CAD build for the part. Positions are in the model's coordinates, mm. A direction names the side the tool comes from. Coordinates: 2 decimals unless noted, no trailing zeros. Order: outer loops, then holes, each group sorted by start corner. A loop starts at its lowest first (then second) coordinate and runs counter-clockwise, first axis right, second up. Notation, with made-up numbers: (77.5, 72.25) - (136.5, 72.25) arc R15 cw to (136.5, 97.25) - close; hole circle Ø2 at (-0.75, 12). An arc over 180 degrees is marked (long way). Write each question's results on one line, items separated by ' | '. Start each with the question number.
Q1. Wall check: probe 1 along Y at (x, z) = (0, 57); probe 2 along Z at (x, y) = (-16.5, -14); probe 3 along X at (y, z) = (15.5, 40). Give the ranges that are in metal, low to high.
Q2. Pin check, flat tips, straight feed: P1, Ø10, axis at y = -24, z = 52.5, coming from the +X side; P2, Ø2, axis at y = 29.5, z = 26, coming from the -X side; P3, Ø8, axis at y = 28, z = 12, coming from the +X side. Stop position of each tip, or through.
Q3. Which spindle directions (+Z, -Z, +X, -X, +Y, -Y) get a long thin tool onto all of the face, cutting with end or side? Do faces 4 (the flat face through (-1, 1, 0)), 5 (the cylindrical face through (-5.012, 38.172, 47.109)), 6 (the flat face through (-4.447, -38.864, 46.097)). Say none if no direction does.
Q4. Band-saw the part on B-B, the plane y = 0. Write the cut outline in (x, z), then the cut area to 3 significant figures.
Q5. Band-saw the part on A-A, the plane x = 9.5. Write the cut outline in (y, z), then the cut area to 3 significant figures.
Q6. Pull direction Y, two halves, no side cores. Call faces 1 (the flat face through (7.62, -38.18, 40.33)), 2 (the flat face through (-1, 1, 3)), 3 (the cylindrical face through (-5.21, 39.66, 44.37)): released by +Y, released by -Y, zero draft, split by the parting line, or undercut.
Q7. Band-saw the part on D-D, the plane x = 0. Write the cut outline in (y, z).
Q8. Band-saw the part on C-C, the plane z = 82. Write the cut outline in (x, y), then the cut area to 3 significant figures.
```python
from build123d import *

# Parameters (mm, degrees)
SKETCH_R        = 40
PAD_DEPTH       = 90
SKETCH001_R     = 38.5
POCKET_DEPTH    = 87
POCKET001_DEPTH = 50


with BuildPart() as part:
    # Sketch → Pad (new body)
    with BuildSketch(Plane.XY):
        Circle(SKETCH_R)
    extrude(amount=PAD_DEPTH)

    # Sketch001 (on Face3 of Pad) → Pocket (cut)
    with BuildSketch(Plane.XY.offset(90)):
        Circle(SKETCH001_R)
    extrude(amount=-POCKET_DEPTH, mode=Mode.SUBTRACT)

    # Sketch002 → Pocket001 (cut)
    with BuildSketch(Plane.XZ.offset(45)):
        Polygon((-19.683228, 16.045872), (10.932937, 76.430139), (22.858825, 70.387448), (-7.758954, 10), align=None)
    extrude(amount=-POCKET001_DEPTH, mode=Mode.SUBTRACT)


solid = part.part
```
Results below:
1) probe 1: y = -40 to -38.5, 38.5 to 40 | probe 2: z = 0 to 3 | probe 3: x = -36.87 to -35.24, 35.24 to 36.87
2) P1: stops at x = 35.2 | P2: stops at x = -28.07 | P3: stops at x = 32
3) face 4: -Z, +X, -X, +Y, -Y | face 5: +Z | face 6: -Y
4) outline: (-40, 0) - (40, 0) - (40, 90) - (38.5, 90) - (38.5, 3) - (-38.5, 3) - (-38.5, 90) - (-40, 90) - close | area: 501 mm²
5) outline: (-38.86, 0) - (38.86, 0) - (38.86, 90) - (37.31, 90) - (37.31, 3) - (-37.31, 3) - (-37.31, 44.04) - (-38.86, 44.04) - close; (-38.86, 73.6) - (-37.31, 73.6) - (-37.31, 90) - (-38.86, 90) - close | area: 456 mm²
6) face 1: zero draft | face 2: undercut | face 3: split by the parting line
7) outline: (-40, 0) - (40, 0) - (40, 90) - (38.5, 90) - (38.5, 3) - (-38.5, 3) - (-38.5, 25.3) - (-40, 25.3) - close; (-40, 54.87) - (-38.5, 54.87) - (-38.5, 90) - (-40, 90) - close
8) outline: circle Ø80 at (0, 0); hole circle Ø77 at (0, 0) | area: 370 mm²
